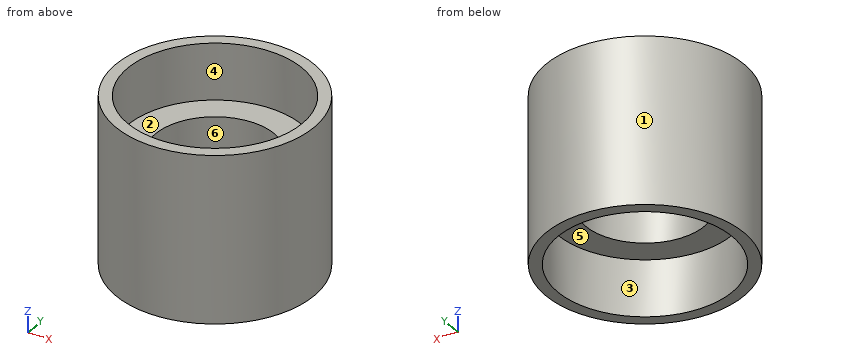
from build123d import *

# Parameters (mm, degrees)
CYLINDER003_R     = 11
CYLINDER003_DEPTH = 7.1
CYLINDER002_R     = 11
CYLINDER002_DEPTH = 7.1
CYLINDER001_R     = 7.5
CYLINDER001_DEPTH = 50
CYLINDER_R        = 12.5
CYLINDER_DEPTH    = 21


with BuildPart() as cylindre003:
    # Cylinder003 → Cylinder003 (new body)
    with BuildSketch(Plane.XY.offset(13.91)):
        Circle(CYLINDER003_R)
    extrude(amount=CYLINDER003_DEPTH)


with BuildPart() as cylindre002:
    # Cylinder002 → Cylinder002 (new body)
    with BuildSketch(Plane.XY.offset(-0.0001)):
        Circle(CYLINDER002_R)
    extrude(amount=CYLINDER002_DEPTH)


with BuildPart() as cylindre001:
    # Cylinder001 → Cylinder001 (new body)
    with BuildSketch(Plane.XY.offset(-11)):
        Circle(CYLINDER001_R)
    extrude(amount=CYLINDER001_DEPTH)


with BuildPart() as cut002:
    # Cylinder → Cylinder (new body)
    with BuildSketch(Plane.XY):
        Circle(CYLINDER_R)
    extrude(amount=CYLINDER_DEPTH)

    # Cut: cut Cylindre001
    add(cylindre001.part, mode=Mode.SUBTRACT)

    # Cut001: cut Cylindre002
    add(cylindre002.part, mode=Mode.SUBTRACT)

    # Cut002: cut Cylindre003
    add(cylindre003.part, mode=Mode.SUBTRACT)


solid = cut002.part
Input: part model. Units: mm. Frame: model coordinates. Face numbers are marked on the shaded views. A direction names the side the tool comes from. Coordinates: 2 decimals unless noted, no trailing zeros. Order: outer loops, then holes, each group sorted by start corner. A loop starts at its lowest first (then second) coordinate and runs counter-clockwise, first axis right, second up. Notation, with made-up numbers: M 38,81.5 L 63,81.5 A23 ccw 63,118.5 Z; hole C 25.5,76 d11. An arc over 180 degrees is marked long. Answer as CSV lines item,"result".
1. Section C-C (z = 8). Return the cut outline in (x, y).
Reported:
outline,"C 0,0 d25; hole C 0,0 d15"
2. First-contact query: P1, Ø8, axis at x = 6.5, z = 7, coming from the +Y side; P2, Ø1.5, axis at x = 2.5, z = 7.5, coming from the -Y side; P3, Ø1.5, axis at x = 5, z = 8.5, coming from the -Y side; P4, Ø6.5, axis at x = -1, y = 1, coming from the -Z side. Flat tips, straight axial feed; report the tip coordinate or a pass-through.
Reported:
P1,"y = 12.25"
P2,"y = -12.38"
P3,"y = -11.76"
P4,"through"
3. Material intervals for line 1 (Y direction, x = 0, z = 15.75); line 2 (Z direction, x = -9, y = -3.5); line 3 (X direction, y = 4, z = 6.5), sorted ascending. Write a range as from..to.
Reported:
line 1,"-12.5..-11, 11..12.5"
line 2,"7.1..13.91"
line 3,"-11.84..-10.25, 10.25..11.84"
4. Section D-D (y = 8). Return the cut outline in (x, z).
Reported:
outline,"M -9.6,0 L -7.55,0 L -7.55,7.1 L 7.55,7.1 L 7.55,0 L 9.6,0 L 9.6,21 L 7.55,21 L 7.55,13.91 L -7.55,13.91 L -7.55,21 L -9.6,21 Z"
5. Access query for the marked faces 4, 5 and 6. Directions: +Z, -Z, +X, -X, +Y, -Y. A direction counts if a zero-diameter tool reaches every point of the face in a straight line with its end or side. Return the directions, or none.
Reported:
face 4,"+Z"
face 5,"-Z"
face 6,"+Z, -Z"
6. Pull-direction query (X, two-part tool) for the marked faces 1, 2 and 3; classes: released by +X, released by -X, zero draft, split by the parting line, or undercut.
Reported:
face 1,"split by the parting line"
face 2,"undercut"
face 3,"undercut"
7. Section A-A (x = 0). Return the cut outline in (y, z), then the cut area to 3 significant figures.
Reported:
outline,"M -12.5,0 L -11,0 L -11,7.1 L -7.5,7.1 L -7.5,13.91 L -11,13.91 L -11,21 L -12.5,21 Z; M 7.5,7.1 L 11,7.1 L 11,0 L 12.5,0 L 12.5,21 L 11,21 L 11,13.91 L 7.5,13.91 Z"
area,"111 mm2"
